Input: dimensioned drawing with shaded views. Units: mm. Origin: part minimum x, y, z. A direction names the side the tool comes from. Coordinates: 2 decimals unless noted, no trailing zeros. Order: outer loops, then holes, each group sorted by start corner. A loop starts at its lowest first (then second) coordinate and runs counter-clockwise, first axis right, second up. Notation, with made-up numbers: (18.5, -7) -> (31.5, -7) arc R22 cw to (31.5, 3) -> close; hole circle Ø2 at (82, 40). An arc over 180 degrees is marked (long way). Write item = value, one per line. Start each with the question number.
Item 1: Section query B-B (y = 21.5). Output: boundary loops of the cut face in (x, z), then the cut area to 3 significant figures.
Item 2: Section query A-A (z = 3). Output: boundary loops of the cut face in (x, y), then the cut area to 3 significant figures.
Item 3: Contact query for flat-ended pins moving along their axis: pin 1 (12 mm diameter, centred on x = 15, z = 3.5, fed in from +Y); pin 2 (10 mm diameter, centred on x = 16, z = 16, fed in from +Y); pin 3 (7.5 mm diameter, centred on x = 4.5, z = 12, fed in from +Y). Output: stop coordinate, or through.
Item 4: Set-up query: the marked faces 1 and 2. Return all of +Z, -Z, +X, -X, +Y, -Y with unobstructed straight access to the full face (end or side cutting, diameter ignored); none if empty.
Item 5: Section query D-D (z = 5.75). Output: boundary loops of the cut face in (x, y).
Item 6: Ray query, line 1 along X through (y, z) = (18, 3.5); line 2 along Y through (x, z) = (8.75, 20.5); line 3 along Y through (x, z) = (25.5, 8). Return the intervals inside material, ascending. Write a range as [from, to].
Item 7: Section query C-C (x = 8.25). Output: boundary loops of the cut face in (y, z).
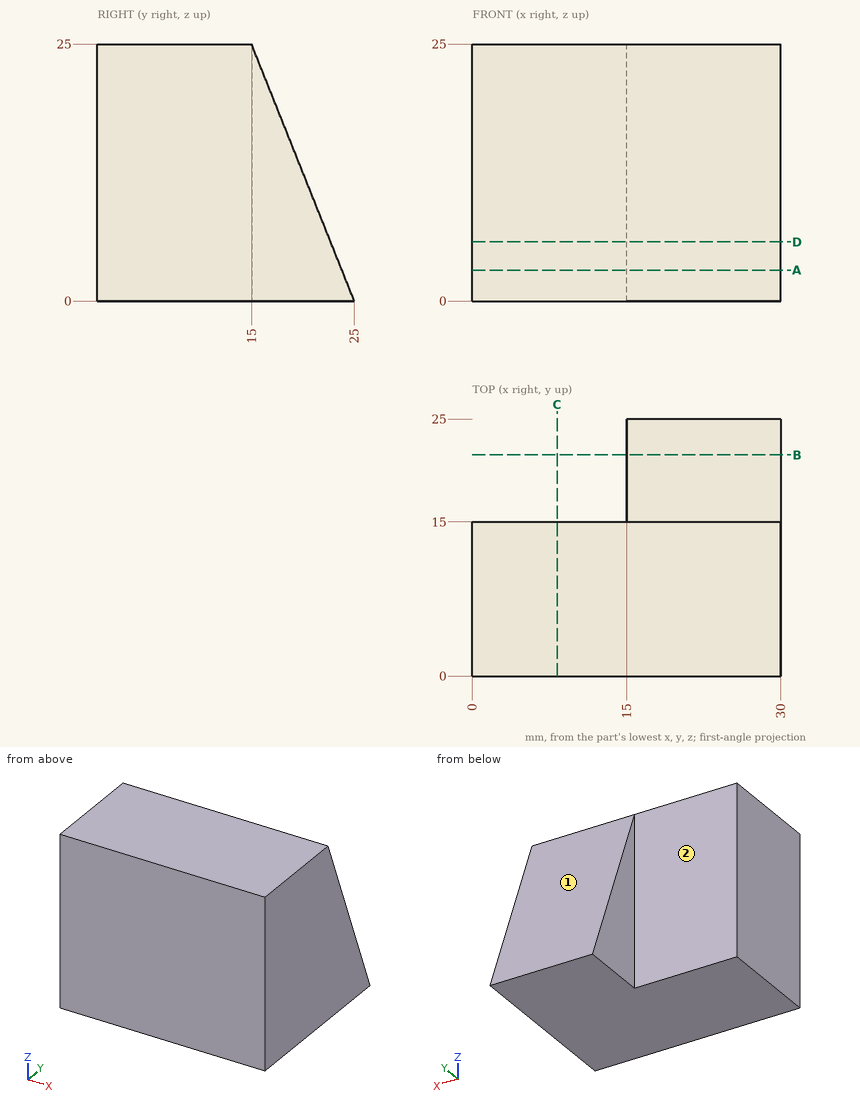
Computed:
q1.outline = (15, 0) -> (30, 0) -> (30, 8.75) -> (15, 8.75) -> close
q1.area = 131 mm^2
q2.outline = (0, 0) -> (30, 0) -> (30, 23.8) -> (15, 23.8) -> (15, 15) -> (0, 15) -> close
q2.area = 582 mm^2
q3.pin_1 = 25
q3.pin_2 = 20.6
q3.pin_3 = 15
q4.face_1 = +Z, +X, -X, +Y
q4.face_2 = +Z, -Z, -X, +Y
q5.outline = (0, 0) -> (30, 0) -> (30, 22.7) -> (15, 22.7) -> (15, 15) -> (0, 15) -> close
q6.line_1 = [15, 30]
q6.line_2 = [0, 15]
q6.line_3 = [0, 21.8]
q7.outline = (0, 0) -> (15, 0) -> (15, 25) -> (0, 25) -> close
